Verification items for the finished model (mm, model axes). A direction names the side the tool comes from. Round coordinates to 2 decimals unless told otherwise and drop trailing zeros. Write each loop counter-clockwise with the first axis right and the second up, starting at its lowest first coordinate (ties: lowest second). Pieces come first, ordered by that corner, then holes. Notation, with made-up numbers: M -21.5,27.5 L -8.5,27.5 A23 ccw -8.5,66.5 Z; hole C 89,34.5 d3. An arc over 180 degrees is marked long. One line per question, with ' | ' between items.
from build123d import *

# Parameters (mm, degrees)
SKETCH1_W               = 90
SKETCH1_H               = 70
BASE_PLATE_DEPTH        = 6
SKETCH4_W               = 86
SKETCH4_H               = 66
SKETCH4_W_2             = 80
SKETCH4_H_2             = 60
SEALANT_CUT_OUTER_DEPTH = 5
SEALANT_CUT_OUTER_TAPER = 35
SKETCH7_R               = 2
SCRE_CUT_DEPTH          = 5
SKETCH12_W              = 64
SKETCH12_H              = 52
SKETCH12_W_2            = 58
SKETCH12_H_2            = 46
SEALANT_CUT_INNER_DEPTH = 3
SEALANT_CUT_INNER_TAPER = 35
SKETCH14_W              = 65
SKETCH14_H              = 45
BASE_BLOCK_DEPTH        = 14
SKETCH13_W              = 48
SKETCH13_H              = 36
DRAIN_DEPTH             = 16
DRAIN_DRAFT             = -40
SKETCH15_R              = 9.75
HOSE_CONNECTOR_DEPTH    = 20
SKETCH16_R              = 7.25
DRAIN_HOLE_DEPTH        = 70.641941443
FILLET1_R               = 10
FILLET2_R               = 10
FILLET3_R               = 10
FILLET4_R               = 10
FILLET5_R               = 10


with BuildPart() as part:
    # Sketch1 → Base Plate (new body)
    with BuildSketch(Plane(origin=(0, 0, 0), x_dir=(1, 0, 0), z_dir=(0, 1, 0))):
        Rectangle(SKETCH1_W, SKETCH1_H)
    extrude(amount=BASE_PLATE_DEPTH)

    # Sketch4 → Sealant Cut - Outer (cut)
    with BuildSketch(Plane(origin=(0, 6, 0), x_dir=(1, 0, 0), z_dir=(0, 1, 0))):
        Rectangle(SKETCH4_W, SKETCH4_H)
        Rectangle(SKETCH4_W_2, SKETCH4_H_2, mode=Mode.SUBTRACT)
    extrude(amount=-SEALANT_CUT_OUTER_DEPTH, taper=SEALANT_CUT_OUTER_TAPER, mode=Mode.SUBTRACT)

    # Sketch7 → Scre Cut (cut)
    with BuildSketch(Plane(origin=(0, 6, 0), x_dir=(1, 0, 0), z_dir=(0, 1, 0))):
        with Locations(Location((-36, 26, 0), (0, 0, 270))):
            Circle(SKETCH7_R)
        with Locations(Location((-36, -26, 0), (0, 0, 90))):
            Circle(SKETCH7_R)
        with Locations(Location((36, -26, 0), (0, 0, 270))):
            Circle(SKETCH7_R)
        with Locations(Location((36, 26, 0), (0, 0, 90))):
            Circle(SKETCH7_R)
    extrude(amount=-SCRE_CUT_DEPTH, mode=Mode.SUBTRACT)

    # Sketch12 → Sealant Cut - Inner (cut)
    with BuildSketch(Plane(origin=(0, 6, 0), x_dir=(1, 0, 0), z_dir=(0, 1, 0))):
        Rectangle(SKETCH12_W, SKETCH12_H)
        Rectangle(SKETCH12_W_2, SKETCH12_H_2, mode=Mode.SUBTRACT)
    extrude(amount=-SEALANT_CUT_INNER_DEPTH, taper=SEALANT_CUT_INNER_TAPER, mode=Mode.SUBTRACT)

    # Sketch14 → Base Block (add)
    with BuildSketch(Plane.XZ):
        Rectangle(SKETCH14_W, SKETCH14_H)
    extrude(amount=BASE_BLOCK_DEPTH)


with BuildPart() as drain_tool:
    # Sketch13 → Drain (with draft: the straight prism first)
    with BuildSketch(Plane(origin=(0, 6, 0), x_dir=(1, 0, 0), z_dir=(0, 1, 0))):
        Rectangle(SKETCH13_W, SKETCH13_H)
    extrude(amount=-DRAIN_DEPTH)
    # Drain: the draft: its side faces are tilted about the plane it starts from
    drain_sides = [drain_tool.faces().sort_by_distance(p)[0] for p in [
        (-24, -2, 0),
        (0, -2, 18),
        (24, -2, 0),
        (0, -2, -18),
    ]]
    draft(drain_sides, Plane(origin=(0, 6, 0), x_dir=(1, 0, 0), z_dir=(0, 1, 0)), DRAIN_DRAFT)


with BuildPart() as part_1:
    add(part.part)

    # Drain: cut by drain_tool
    add(drain_tool.part, mode=Mode.SUBTRACT)

    # Sketch15 → Hose connector (add)
    with BuildSketch(Plane.XZ.offset(14)):
        with Locations(Location((0, 0, 0), (0, 0, 270))):
            Circle(SKETCH15_R)
    extrude(amount=HOSE_CONNECTOR_DEPTH)

    # Sketch16 → Drain Hole (cut, through all)
    with BuildSketch(Plane.XZ.offset(34)):
        with Locations(Location((0, 0, 0), (0, 0, 270))):
            Circle(SKETCH16_R)
    extrude(amount=-DRAIN_HOLE_DEPTH, mode=Mode.SUBTRACT)

    # Fillet1
    fillet1_edges = [part_1.edges().sort_by_distance(p)[0] for p in [
        (-32.5, -7, -22.5),
    ]]
    fillet(fillet1_edges, radius=FILLET1_R)

    # Fillet2
    fillet2_edges = [part_1.edges().sort_by_distance(p)[0] for p in [
        (32.5, -7, -22.5),
    ]]
    fillet(fillet2_edges, radius=FILLET2_R)

    # Fillet3
    fillet3_edges = [part_1.edges().sort_by_distance(p)[0] for p in [
        (32.5, -7, 22.5),
    ]]
    fillet(fillet3_edges, radius=FILLET3_R)

    # Fillet4
    fillet4_edges = [part_1.edges().sort_by_distance(p)[0] for p in [
        (-32.5, -7, 22.5),
    ]]
    fillet(fillet4_edges, radius=FILLET4_R)

    # Srew Heads cone 1 section (through the dimple's axis) → Srew Heads (revolve, cut)
    with BuildSketch(Plane(origin=(-36, 0, -26), x_dir=(0, 0, -1), z_dir=(1, 0, 0))):
        Polygon((0, 0), (2.75, 0), (0, 2.75), align=None)
    revolve(axis=Axis((-36, 0, -26), (0, 1, 0)), mode=Mode.SUBTRACT)

    # Srew Heads cone 2 section (through the dimple's axis) → Srew Heads cone 2 (revolve, cut)
    with BuildSketch(Plane(origin=(-36, 0, 26), x_dir=(0, 0, -1), z_dir=(1, 0, 0))):
        Polygon((0, 0), (2.75, 0), (0, 2.75), align=None)
    revolve(axis=Axis((-36, 0, 26), (0, 1, 0)), mode=Mode.SUBTRACT)

    # Srew Heads cone 3 section (through the dimple's axis) → Srew Heads cone 3 (revolve, cut)
    with BuildSketch(Plane(origin=(36, 0, 26), x_dir=(0, 0, -1), z_dir=(1, 0, 0))):
        Polygon((0, 0), (2.75, 0), (0, 2.75), align=None)
    revolve(axis=Axis((36, 0, 26), (0, 1, 0)), mode=Mode.SUBTRACT)

    # Srew Heads cone 4 section (through the dimple's axis) → Srew Heads cone 4 (revolve, cut)
    with BuildSketch(Plane(origin=(36, 0, -26), x_dir=(0, 0, -1), z_dir=(1, 0, 0))):
        Polygon((0, 0), (2.75, 0), (0, 2.75), align=None)
    revolve(axis=Axis((36, 0, -26), (0, 1, 0)), mode=Mode.SUBTRACT)

    # Fillet5
    fillet5_edges = [part_1.edges().sort_by_distance(p)[0] for p in [
        (0, -14, -22.5),
        (-29.571067812, -14, -19.571067812),
        (32.5, -14, 0),
        (29.571067812, -14, -19.571067812),
        (0, -14, 22.5),
        (29.571067812, -14, 19.571067812),
        (-32.5, -14, 0),
        (-29.571067812, -14, 19.571067812),
    ]]
    fillet(fillet5_edges, radius=FILLET5_R)


solid = part_1.part
1. Tool access check on faces 1 (the face through (0, -2, -22.5)), 2 (the face through (9.667, -23.86, 1.269)), 3 (the face through (32.5, -2, 0)), 4 (the face through (-0.336, -0.11, 12.873)), 5 (the face through (7.3, -34, 1.5)). Record the directions out of +Z, -Z, +X, -X, +Y, -Y that give a thin tool (end or side, any length) a straight path to the whole face; none if there is none.
Results:
face 1: -Z, +X, -X, -Y | face 2: -Y | face 3: +Z, -Z, +X, -Y | face 4: +Y | face 5: +Z, -Z, +X, -X, -Y
2. Mould release check, pull along X, two halves, no side actions. Record for faces 6 (the face through (-18.873, -0.11, 0.252)), 7 (the face through (-45, 3, 0)), 8 (the face through (0, -2, 22.5)): pulls with the +X half, pulls with the -X half, needs draft (parallel to the pull), parting line crosses it, or undercut.
Results:
face 6: undercut | face 7: pulls with the -X half | face 8: needs draft
3. Section check B-B, the plane y = -18. Record the cut outline in (x, z), then the cut area to 3 significant figures.
Results:
outline: C 0,0 d19.5; hole C 0,0 d14.5 | area: 134 mm2
4. Thickness scan on line 1 (X direction, y = 2.1, z = -26); line 2 (X direction, y = 4, z = 26); line 3 (X direction, y = -23, z = -4). Record the ranges inside material, lowest first.
Results:
line 1: x = -45 to -38, -34 to 34, 38 to 45 | line 2: x = -45 to -41.6, -41.4 to -38, -34 to 34, 38 to 41.4, 41.6 to 45 | line 3: x = -8.89 to -6.05, 6.05 to 8.89
5. Go/stop test with flat-tipped pins: P1, Ø10, axis at x = -14, y = -13.5, coming from the -Z side; P2, Ø8, axis at y = -16, z = 1.5, coming from the +X side; P3, Ø1, axis at x = 7.5, y = -17, coming from the -Z side. Record where each tip stops, or that it passes through.
Results:
P1: stops at z = -21.43 | P2: stops at x = 28.5 | P3: stops at z = -6.79
6. Section check A-A, the plane x = -36. Count the separate pieces of the cut face and the enclosed holes in it, then the cut area to 3 significant figures.
Results:
separate pieces: 3 | enclosed holes: 0 | area: 365 mm2
